```python
from build123d import *

# Parameters (mm, degrees)
BOSS_EXTRUDE1_DEPTH     = 10
CUT_EXTRUDE1_DEPTH      = 48.916594203
CUT_EXTRUDE1_DEPTH_BACK = 48.916594203
SKETCH2_R               = 1.65
CHAMFER1_SIZE           = 1.6
FILLET1_R               = 5
FILLET2_R               = 5


with BuildPart() as part:
    # Sketch1 → Boss-Extrude1 (new body)
    with BuildSketch(Plane.XY):
        Polygon((0, 0), (0, 5), (-14, 5), (-14, 25), (0, 25), (0, 30), (-36, 30), (-36, 25), (-22, 25), (-22, 5), (-36, 5), (-36, 0), align=None)
    extrude(amount=BOSS_EXTRUDE1_DEPTH)

    # Sketch2 → Cut-Extrude1 (cut, two sides: drawn at the far end of the back side and taken through both)
    with BuildSketch(Plane(origin=(0, 30, 0), x_dir=(1, 0, 0), z_dir=(0, 1, 0)).offset(-CUT_EXTRUDE1_DEPTH_BACK)):
        with Locations(Location((-32, -5, 0), (0, 0, 180))):
            Circle(SKETCH2_R)
        with Locations(Location((-4, -5, 0), (0, 0, 180))):
            Circle(SKETCH2_R)
    extrude(amount=CUT_EXTRUDE1_DEPTH + CUT_EXTRUDE1_DEPTH_BACK, mode=Mode.SUBTRACT)

    # Chamfer1
    chamfer1_edges = [part.edges().sort_by_distance(p)[0] for p in [
        (-30.35, 5, 5),
        (-2.35, 5, 5),
    ]]
    chamfer(chamfer1_edges, length=CHAMFER1_SIZE)

    # Fillet1
    fillet1_edges = [part.edges().sort_by_distance(p)[0] for p in [
        (-22, 5, 5),
        (-22, 25, 5),
        (-14, 25, 5),
        (-14, 5, 5),
    ]]
    fillet(fillet1_edges, radius=FILLET1_R)

    # Fillet2
    fillet2_edges = [part.edges().sort_by_distance(p)[0] for p in [
        (0, 27.5, 10),
        (0, 27.5, 0),
        (0, 2.5, 0),
        (0, 2.5, 10),
        (-36, 2.5, 0),
        (-36, 2.5, 10),
        (-36, 27.5, 0),
        (-36, 27.5, 10),
    ]]
    fillet(fillet2_edges, radius=FILLET2_R - 0.0001)  # a hair under: the kernel refuses the full size


solid = part.part
```
Check sheet for the modelled part. Datum: model origin and axes. Units: mm. A direction names the side the tool comes from. Coordinates: 2 decimals unless noted, no trailing zeros. Loops run counter-clockwise (first coordinate to the right, second up) from the corner with the lowest first, then second, coordinate; pieces in that order, holes last.
1) Sectioned sample at C-C (x = -32). Record the boundary of the cut face in (y, z), and give its area (3 significant figures).
2) Material ranges on probe 1 along X at (y, z) = (0.8, 5); probe 2 along X at (y, z) = (1.75, 6.5); probe 3 along Y at (x, z) = (-27, 4), recorded low to high.
3) Access from +Z, -Z, +X, -X, +Y, -Y to the whole of each face (thin tool, end or side, straight path). Record for faces 1 (the face through (-23, 7, 5)), 2 (the face through (-1, 3, 8)), 3 (the face through (-13, 23, 5)).
4) Release check for a two-part mould opening along Y. For faces 4 (the face through (-18, 0, 5)), 5 (the face through (-34, 2, 9)), 6 (the face through (-28, 5, 5)) record: released by +Y, released by -Y, zero draft, split by the parting line, or undercut.
5) Sectioned sample at B-B (x = -25.5). Record the boundary of the cut face in (y, z), and give its area (3 significant figures).
6) Sectioned sample at A-A (y = 4). Count the separate pieces of the cut face and the enclosed holes in it, and give its area (3 significant figures).
7) Gauge pin test, flat ends, axial feed: pin 1 (2.5 mm diameter, centred on x = -32, z = 5, fed in from +Y); pin 2 (3 mm diameter, centred on y = 13, z = 5, fed in from -X); pin 3 (2 mm diameter, centred on y = 21.5, z = 9, fed in from +X). Record the tip position at first contact, or that the pin passes through.
Check sheet entries:
1. outline: (0, 0.1) - (5, 0.1) - (5, 1.75) - (3.4, 3.35) - (0, 3.35) - close; (0, 6.65) - (3.4, 6.65) - (5, 8.25) - (5, 9.9) - (0, 9.9) - close; (25, 0.1) - (30, 0.1) - (30, 3.35) - (25, 3.35) - close; (25, 6.65) - (30, 6.65) - (30, 9.9) - (25, 9.9) - close
1. area: 62.4 mm2
2. probe 1: x = -36 to -33.65, -30.35 to -5.65, -2.35 to 0
2. probe 2: x = -35.77 to -32.69, -31.31 to -4.69, -3.31 to -0.23
2. probe 3: y = 0 to 5, 25 to 30
3. face 1: +Z, -Z, -X
3. face 2: +Z, +X, +Y, -Y
3. face 3: +Z, -Z, +X
4. face 4: released by -Y
4. face 5: zero draft
4. face 6: undercut
5. outline: (0, 0) - (5.23, 0) - (5.23, 10) - (0, 10) - close; (24.77, 0) - (30, 0) - (30, 10) - (24.77, 10) - close
5. area: 105 mm2
6. separate pieces: 1
6. enclosed holes: 2
6. area: 307 mm2
7. pin 1: passes through
7. pin 2: stops at x = -22
7. pin 3: stops at x = -13.33
